Source: CAD feature listing. Evaluate the final solid. Frame: model axes, mm. A direction names the side the tool comes from. Coordinates: 2 decimals unless noted, no trailing zeros. Order: outer loops, then holes, each group sorted by start corner. A loop starts at its lowest first (then second) coordinate and runs counter-clockwise, first axis right, second up.
```python
from build123d import *

# Parameters (mm, degrees)
SKETCH1_W           = 762
SKETCH1_H           = 12.7
BOSS_EXTRUDE1_DEPTH = 609.6
SKETCH2_W           = 12.7
SKETCH2_H           = 609.6
BOSS_EXTRUDE2_DEPTH = 76.2
SKETCH3_OUTSIDE_W   = 1136.21
SKETCH3_OUTSIDE_H   = 831.41
CUT_EXTRUDE1_DEPTH  = 12.7
SKETCH6_W           = 56.167651581
SKETCH6_H           = 12.7
SKETCH6_W_2         = 683.835303162
CUT_EXTRUDE2_DEPTH  = 12.7
CUT_EXTRUDE5_DEPTH  = 12.7
SKETCH7_W           = 12.7
SKETCH7_H           = 88.9
CUT_EXTRUDE3_DEPTH  = 12.7
SKETCH10_R          = 28.575
CUT_EXTRUDE4_DEPTH  = 763.105825985
BOSS_EXTRUDE5_START = -88.9
SKETCH11_W          = 12.7
SKETCH11_H          = 12.7
BOSS_EXTRUDE5_DEPTH = 88.9
SKETCH12_W          = 56.167651581
SKETCH12_H          = 12.7
SKETCH12_W_2        = 683.835303162
BOSS_EXTRUDE6_DEPTH = 12.7


with BuildPart() as part:
    # Sketch1 → Boss-Extrude1 (new body)
    with BuildSketch(Plane(origin=(0, 0, 0), x_dir=(1, 0, 0), z_dir=(0, 1, 0))):
        with Locations((0, -653.561357684)):
            Rectangle(SKETCH1_W, SKETCH1_H)
    extrude(amount=BOSS_EXTRUDE1_DEPTH)

    # Sketch2 → Boss-Extrude2 (add)
    with BuildSketch(Plane(origin=(381, 0, 0), x_dir=(0, 0, -1), z_dir=(1, 0, 0))):
        with Locations((-653.561357684, 304.8)):
            Rectangle(SKETCH2_W, SKETCH2_H)
    boss_extrude2 = extrude(amount=BOSS_EXTRUDE2_DEPTH)

    # Mirror1: Boss-Extrude2 across plane
    add(boss_extrude2.mirror(Plane(origin=(0, 0, 0), x_dir=(0, 0, 1), z_dir=(1, 0, 0))))

    # Sketch3 outside → Cut-Extrude1 (cut)
    with BuildSketch(Plane.XY.offset(659.911357684)):
        with Locations((0, 304.8)):
            Rectangle(SKETCH3_OUTSIDE_W, SKETCH3_OUTSIDE_H)
        Polygon((366.335303163, 609.6), (-366.335303163, 609.6), (-366.335303163, 533.4), (-388.332348419, 533.4), (-388.332348419, 609.6), (-457.2, 609.6), (-457.2, 457.2), (-366.335303163, 457.2), (-366.335303163, 304.8), (-388.332348419, 304.8), (-388.332348419, 381), (-457.2, 381), (-457.2, 228.6), (-366.335303163, 228.6), (-366.335303163, 76.2), (-388.332348419, 76.2), (-388.332348419, 152.4), (-457.2, 152.4), (-457.2, 0), (457.2, 0), (457.2, 152.4), (388.332348419, 152.4), (388.332348419, 76.2), (366.335303163, 76.2), (366.335303163, 228.6), (457.2, 228.6), (457.2, 381), (388.332348419, 381), (388.332348419, 304.8), (366.335303163, 304.8), (366.335303163, 457.2), (457.2, 457.2), (457.2, 609.6), (388.332348419, 609.6), (388.332348419, 533.4), (366.335303163, 533.4), align=None, mode=Mode.SUBTRACT)
    extrude(amount=-CUT_EXTRUDE1_DEPTH, mode=Mode.SUBTRACT)

    # Sketch6 → Cut-Extrude2 (cut)
    with BuildSketch(Plane(origin=(0, 609.6, 0), x_dir=(1, 0, 0), z_dir=(0, 1, 0))):
        with Locations((-416.41617421, -653.561357684)):
            Rectangle(SKETCH6_W, SKETCH6_H)
        with Locations((0, -653.561357684)):
            Rectangle(SKETCH6_W_2, SKETCH6_H)
        with Locations((416.41617421, -653.561357684)):
            Rectangle(SKETCH6_W, SKETCH6_H)
    cut_extrude2 = extrude(amount=-CUT_EXTRUDE2_DEPTH, mode=Mode.SUBTRACT)

    # Sketch14 → Cut-Extrude5 (cut)
    with BuildSketch(Plane.XY.offset(659.911357684)):
        Polygon((-388.332348419, 457.2), (-457.2, 501.65), (-457.2, 457.2), align=None)
        Polygon((-388.332348419, 381), (-457.2, 336.55), (-457.2, 381), align=None)
        Polygon((-388.332348419, 152.4), (-457.2, 107.95), (-457.2, 152.4), align=None)
        Polygon((457.2, 152.4), (388.332348419, 152.4), (457.2, 107.95), align=None)
        Polygon((457.2, 381), (388.332348419, 381), (457.2, 336.55), align=None)
        Polygon((457.2, 457.2), (388.332348419, 457.2), (457.2, 501.65), align=None)
        Polygon((-457.2, 273.05), (-388.332348419, 228.6), (-457.2, 228.6), align=None)
        Polygon((388.332348419, 228.6), (457.2, 228.6), (457.2, 273.05), align=None)
    extrude(amount=-CUT_EXTRUDE5_DEPTH, mode=Mode.SUBTRACT)

    # Sketch7 → Cut-Extrude3 (cut)
    with BuildSketch(Plane.XY.offset(659.911357684)):
        with Locations((154.820606325, 552.45)):
            Rectangle(SKETCH7_W, SKETCH7_H)
        with Locations((-154.820606325, 552.45)):
            Rectangle(SKETCH7_W, SKETCH7_H)
    cut_extrude3 = extrude(amount=-CUT_EXTRUDE3_DEPTH, mode=Mode.SUBTRACT)

    # Mirror2: Cut-Extrude2, Cut-Extrude3 across plane
    add(cut_extrude2.mirror(Plane(origin=(0, 304.8, 0), x_dir=(0, 0, 1), z_dir=(0, -1, 0))), mode=Mode.SUBTRACT)
    add(cut_extrude3.mirror(Plane(origin=(0, 304.8, 0), x_dir=(0, 0, 1), z_dir=(0, -1, 0))), mode=Mode.SUBTRACT)

    # Sketch10 → Cut-Extrude4 (cut, through all)
    with BuildSketch(Plane.XY.offset(659.911357684)):
        with Locations((-302.835303163, 311.15)):
            Circle(SKETCH10_R)
        with Locations((-302.835303163, 193.675)):
            Circle(SKETCH10_R)
        with Locations((-302.835303163, 76.2)):
            Circle(SKETCH10_R)
        with Locations(Location((-100.945101054, 76.2, 0), (0, 0, 180))):
            Circle(SKETCH10_R)
        with Locations(Location((-100.945101054, 193.675, 0), (0, 0, 180))):
            Circle(SKETCH10_R)
        with Locations(Location((-100.945101054, 311.15, 0), (0, 0, 180))):
            Circle(SKETCH10_R)
        with Locations((-201.890202108, 252.4125)):
            Circle(SKETCH10_R)
        with Locations((-201.890202108, 134.9375)):
            Circle(SKETCH10_R)
        with Locations((100.945101054, 193.675)):
            Circle(SKETCH10_R)
        with Locations((302.835303163, 193.675)):
            Circle(SKETCH10_R)
        with Locations((100.945101054, 311.15)):
            Circle(SKETCH10_R)
        with Locations((302.835303163, 311.15)):
            Circle(SKETCH10_R)
        with Locations((100.945101054, 76.2)):
            Circle(SKETCH10_R)
        with Locations((302.835303163, 76.2)):
            Circle(SKETCH10_R)
        with Locations((0, 134.9375)):
            Circle(SKETCH10_R)
        with Locations((0, 252.4125)):
            Circle(SKETCH10_R)
        with Locations((201.890202108, 252.4125)):
            Circle(SKETCH10_R)
        with Locations((201.890202108, 134.9375)):
            Circle(SKETCH10_R)
        with Locations(Location((302.835303163, 546.1, 0), (0, 0, 180))):
            Circle(SKETCH10_R)
        with Locations(Location((302.835303163, 428.625, 0), (0, 0, 180))):
            Circle(SKETCH10_R)
        with Locations(Location((201.890202108, 369.8875, 0), (0, 0, 180))):
            Circle(SKETCH10_R)
        with Locations(Location((201.890202108, 487.3625, 0), (0, 0, 180))):
            Circle(SKETCH10_R)
        with Locations(Location((100.945101054, 546.1, 0), (0, 0, 180))):
            Circle(SKETCH10_R)
        with Locations(Location((100.945101054, 428.625, 0), (0, 0, 180))):
            Circle(SKETCH10_R)
        with Locations(Location((0, 487.3625, 0), (0, 0, 180))):
            Circle(SKETCH10_R)
        with Locations(Location((0, 369.8875, 0), (0, 0, 180))):
            Circle(SKETCH10_R)
        with Locations((-100.945101054, 428.625)):
            Circle(SKETCH10_R)
        with Locations((-100.945101054, 546.1)):
            Circle(SKETCH10_R)
        with Locations(Location((-201.890202108, 487.3625, 0), (0, 0, 180))):
            Circle(SKETCH10_R)
        with Locations(Location((-302.835303163, 546.1, 0), (0, 0, 180))):
            Circle(SKETCH10_R)
        with Locations(Location((-302.835303163, 428.625, 0), (0, 0, 180))):
            Circle(SKETCH10_R)
        with Locations(Location((-201.890202108, 369.8875, 0), (0, 0, 180))):
            Circle(SKETCH10_R)
    extrude(amount=-CUT_EXTRUDE4_DEPTH, mode=Mode.SUBTRACT)

    # Sketch11 → Boss-Extrude5 (add)
    with BuildSketch(Plane.XZ.offset(-12.7).offset(BOSS_EXTRUDE5_START)):
        with Locations((154.820606325, 653.561357684)):
            Rectangle(SKETCH11_W, SKETCH11_H)
        with Locations((-154.820606325, 653.561357684)):
            Rectangle(SKETCH11_W, SKETCH11_H)
    extrude(amount=BOSS_EXTRUDE5_DEPTH)

    # Sketch12 → Boss-Extrude6 (add)
    with BuildSketch(Plane.XZ.offset(-12.7)):
        with Locations((416.41617421, 653.561357684)):
            Rectangle(SKETCH12_W, SKETCH12_H)
        with Locations((-416.41617421, 653.561357684)):
            Rectangle(SKETCH12_W, SKETCH12_H)
        with Locations((0, 653.561357684)):
            Rectangle(SKETCH12_W_2, SKETCH12_H)
    extrude(amount=BOSS_EXTRUDE6_DEPTH)


solid = part.part
```
1. Contact query for flat-ended pins moving along their axis: P1, Ø4, axis at x = 16.5, z = 654.5, coming from the +Y side; P2, Ø4, axis at y = 135.5, z = 655, coming from the +X side; P3, Ø4, axis at y = 115.5, z = 655, coming from the +X side; P4, Ø4, axis at x = 377.5, z = 651, coming from the -Y side. Output: stop coordinate, or through.
2. Draft query along X for faces 1 (the flat face through (-422.28, 479.11, 653.65)), 2 (the cylindrical face through (-79.884, 174.363, 653.65)), 3 (the flat face through (423.248, 251.136, 653.65)). Return one class per face: +X half, -X half, draft (parallel to the pull), parting line (faces both ways), or undercut.
3. Material intervals for line 1 along Y through (x, z) = (0, 654.5); line 2 along X through (y, z) = (287, 654.5); line 3 along X through (y, z) = (180, 650), sorted ascending.
4. Section query A-A, the plane x = 0. Output: boundary loops of the cut face in (y, z), plus the area to 3 significant figures.
5. Section query B-B, the plane y = 546.1. Count the separate pieces of the cut face and the enclosed holes in it, plus the area to 3 significant figures.
6. Access query for faces 4 (the flat face through (422.28, 479.11, 653.65)), 5 (the cylindrical face through (-87.76, 520.75, 653.65)). Directions: +Z, -Z, +X, -X, +Y, -Y. A direction counts if a zero-diameter tool reaches every point of the face in a straight line with its end or side. Return the directions, or none.
Answer key:
1. P1: stops at y = 596.9
1. P2: stops at x = 417.61
1. P3: stops at x = 448.6
1. P4: stops at y = 0
2. face 1: -X half
2. face 2: undercut
2. face 3: +X half
3. line 1: y = 0 to 106.36, 163.51 to 223.84, 280.99 to 341.31, 398.46 to 458.79, 515.94 to 596.9
3. line 2: x = -457.2 to -318.11, -287.56 to -116.22, -85.67 to 85.67, 116.22 to 287.56, 318.11 to 457.2
3. line 3: x = -366.34 to -327.93, -277.74 to -126.04, -75.85 to 75.85, 126.04 to 277.74, 327.93 to 366.34
4. outline: (0, 647.21) - (106.36, 647.21) - (106.36, 659.91) - (0, 659.91) - close; (163.51, 647.21) - (223.84, 647.21) - (223.84, 659.91) - (163.51, 659.91) - close; (280.99, 647.21) - (341.31, 647.21) - (341.31, 659.91) - (280.99, 659.91) - close; (398.46, 647.21) - (458.79, 647.21) - (458.79, 659.91) - (398.46, 659.91) - close; (515.94, 647.21) - (596.9, 647.21) - (596.9, 659.91) - (515.94, 659.91) - close
4. area: 4,680 mm2
5. separate pieces: 9
5. enclosed holes: 0
5. area: 7,830 mm2
6. face 4: +Z, -Z, +X
6. face 5: +Z, -Z
